```python
from build123d import *

# Parameters (mm, degrees)
SKETCH1_W          = 76.99375
SKETCH1_H          = 203.2
SKETCH1_W_2        = 38.89375
SKETCH1_H_2        = 38.89375
BASE_FLANGE1_DEPTH = 4.7752
FILLET1_R          = 1.5875
FILLET2_R          = 19.05
SKETCH2_W          = 25.4
SKETCH2_H          = 63.5
CUT_EXTRUDE1_DEPTH = 110.917731513


# Sheet-metal steps are written as plain solids
with BuildPart() as part:
    # Sketch1 → Base-Flange1 (new body)
    with BuildSketch(Plane(origin=(0, 0, 0), x_dir=(0, 0, -1), z_dir=(1, 0, 0))):
        with Locations((3.175, 0)):
            Rectangle(SKETCH1_W, SKETCH1_H)
        Rectangle(SKETCH1_W_2, SKETCH1_H_2, mode=Mode.SUBTRACT)
        with BuildLine():
            Line((24.60625, 71.496159823), (24.60625, 46.096159823))
            ThreePointArc((24.60625, 46.096159823), (19.446875, 40.936784823), (14.2875, 46.096159823))
            Line((14.2875, 46.096159823), (14.2875, 71.496159823))
            ThreePointArc((14.2875, 71.496159823), (19.446875, 76.655534823), (24.60625, 71.496159823))
        make_face(mode=Mode.SUBTRACT)
        with BuildLine():
            Line((24.60625, -75.803125), (24.60625, -50.403125))
            ThreePointArc((24.60625, -50.403125), (19.446875, -45.24375), (14.2875, -50.403125))
            Line((14.2875, -50.403125), (14.2875, -75.803125))
            ThreePointArc((14.2875, -75.803125), (19.446875, -80.9625), (24.60625, -75.803125))
        make_face(mode=Mode.SUBTRACT)
    extrude(amount=-BASE_FLANGE1_DEPTH)

    # Fillet1
    fillet1_edges = [part.edges().sort_by_distance(p)[0] for p in [
        (-2.3876, -19.446875, 19.446875),
        (-2.3876, 19.446875, 19.446875),
        (-2.3876, 19.446875, -19.446875),
        (-2.3876, -19.446875, -19.446875),
    ]]
    fillet(fillet1_edges, radius=FILLET1_R)

    # Fillet2
    fillet2_edges = [part.edges().sort_by_distance(p)[0] for p in [
        (-2.3876, -101.6, -41.671875),
        (-2.3876, -101.6, 35.321875),
        (-2.3876, 101.6, 35.321875),
        (-2.3876, 101.6, -41.671875),
    ]]
    fillet(fillet2_edges, radius=FILLET2_R)

    # Sketch2 → Cut-Extrude1 (cut, through all)
    with BuildSketch(Plane.ZY.offset(4.7752)):
        with Locations((22.621875, 69.85)):
            Rectangle(SKETCH2_W, SKETCH2_H)
    extrude(amount=-CUT_EXTRUDE1_DEPTH, mode=Mode.SUBTRACT)


solid = part.part
```
Could you check a few things on this model? Use its own coordinates, in mm. A direction names the side the tool comes from. Round coordinates to 2 decimals unless told otherwise and drop trailing zeros. Order: outer loops, then holes, each group sorted by start corner. A loop starts at its lowest first (then second) coordinate and runs counter-clockwise, first axis right, second up. Notation, with made-up numbers: M 8,-19 L 61,-19 A8 cw 61,-13 Z; hole C -9.5,52.25 d6. An arc over 180 degrees is marked long. One line per question, with ' | ' between items. Start each with the question number.
(1) For P1, Ø2, axis at y = 15, z = -28, coming from the +X side; P2, Ø1.4, axis at x = -1.5, y = 69, coming from the +Z side; P3, Ø1.4, axis at x = -2.5, z = 27.5, coming from the +Y side, each with a flat end and sliding along its axis, tell me the tip position at first contact or that it passes through.
(2) Please list where these lines run through material, in increasing order: line 1 along Y through (x, z) = (-1.4, -20.5); line 2 along Y through (x, z) = (-1.7, -5); line 3 along Y through (x, z) = (-0.6, -22).
(3) Suppose I cut it at D-D on z = 30.5. List the corners of the cut face in (x, y) for me, then the cut area to 3 significant figures.
(4) For faces 1 (the face through (-2.42, -96.17, -35.94)), 2 (the face through (-2, 69, 9.922)), 3 (the face through (-2, -63, -24.606)), which set-ups out of +Z, -Z, +X, -X, +Y, -Y let a thin tool reach every point of the face, with its end or its side?
(5) Suppose I cut it at C-C on x = -2.8. Count the separate pieces of the cut face and the enclosed holes in it, then the cut area to 3 significant figures.
(6) Thinking about a two-plate mould opening in Y: for faces 4 (the face through (-2, 38.1, 22)), 5 (the face through (0, -21, -3)), 6 (the face through (-2, -63, -14.288)), which applies, +Y half, -Y half, draft (parallel to the pull), parting line (faces both ways), or undercut?
(7) Suppose I cut it at B-B on y = 61. List the corners of the cut face in (x, z) for me.
(8) Suppose I cut it at A-A on z = 7.5. List the corners of the cut face in (x, y) for me, then the cut area to 3 significant figures.
Geometry results:
1) P1: x = 0 | P2: z = 9.92 | P3: y = 38.1
2) line 1: -101.6 to -80.85, -45.35 to 41.05, 76.55 to 101.6 | line 2: -101.6 to -19.45, 19.45 to 101.6 | line 3: -101.6 to -80.29, -45.92 to 41.61, 75.98 to 101.6
3) outline: M -4.78,-95.22 L 0,-95.22 L 0,38.1 L -4.78,38.1 Z | area: 637 mm²
4) face 1: -Z, +X, -X, -Y | face 2: +Z, +X, -X, +Y | face 3: +X, -X
5) separate pieces: 1 | enclosed holes: 3 | area: 11,600 mm²
6) face 4: +Y half | face 5: draft | face 6: undercut
7) outline: M -4.78,-41.67 L 0,-41.67 L 0,-24.61 L -4.78,-24.61 Z; M -4.78,-14.29 L 0,-14.29 L 0,9.92 L -4.78,9.92 Z
8) outline: M -4.78,-101.6 L 0,-101.6 L 0,-19.45 L -4.78,-19.45 Z; M -4.78,19.45 L 0,19.45 L 0,101.6 L -4.78,101.6 Z | area: 785 mm²
